```python
from build123d import *

# Parameters (mm, degrees)
SKETCH1_W            = 100
SKETCH1_H            = 40
BOSS_EXTRUDE1_DEPTH  = 150
CUT_EXTRUDE1_DEPTH   = 41
FILLET1_R            = 30
FILLET1_OF_MIRROR1_R = 30


with BuildPart() as part:
    # Sketch1 → Boss-Extrude1 (new body)
    with BuildSketch(Plane.XY):
        with Locations((-50, 20)):
            Rectangle(SKETCH1_W, SKETCH1_H)
    boss_extrude1 = extrude(amount=BOSS_EXTRUDE1_DEPTH)

    # Cut-Sweep1: sweep along a path in Sketch3
    with BuildLine(Plane(origin=(0, 40, 0), x_dir=(1, 0, 0), z_dir=(0, 1, 0))) as cut_sweep1_path:
        Line((-100, -127.5), (-55, -127.5))
        ThreePointArc((-55, -127.5), (-33.786796564, -118.713203436), (-25, -97.5))
        Line((-25, -97.5), (-25, -25))
    # Sketch2 → Cut-Sweep1 (sweep, cut)
    with BuildSketch(Plane.ZY.offset(100)):
        Polygon((135, 40), (120, 40), (120, 20), (112.5, 20), (112.5, 5), (142.5, 5), (142.5, 20), (135, 20), align=None)
    cut_sweep1 = sweep(path=cut_sweep1_path.line, mode=Mode.SUBTRACT)

    # Sketch4 → Cut-Extrude1 (cut, through all)
    with BuildSketch(Plane(origin=(0, 40, 0), x_dir=(1, 0, 0), z_dir=(0, 1, 0))):
        with BuildLine():
            Line((-52.5, -25), (-52.5, 0))
            Line((-52.5, 0), (-100, 0))
            Line((-100, 0), (-100, -100))
            Line((-100, -100), (-55, -100))
            ThreePointArc((-55, -100), (-53.232233047, -99.267766953), (-52.5, -97.5))
            Line((-52.5, -97.5), (-52.5, -25))
        make_face()
    cut_extrude1 = extrude(amount=-CUT_EXTRUDE1_DEPTH, mode=Mode.SUBTRACT)

    # Fillet1
    fillet1_edges = [part.edges().sort_by_distance(p)[0] for p in [
        (-52.5, 20, 0),
    ]]
    fillet(fillet1_edges, radius=FILLET1_R)

    # Mirror1: Boss-Extrude1, Cut-Sweep1, Cut-Extrude1 across plane
    add(boss_extrude1.mirror(Plane(origin=(0, 0, 150), x_dir=(0, 0, 1), z_dir=(-1, 0, 0))))
    add(cut_sweep1.mirror(Plane(origin=(0, 0, 150), x_dir=(0, 0, 1), z_dir=(-1, 0, 0))), mode=Mode.SUBTRACT)
    add(cut_extrude1.mirror(Plane(origin=(0, 0, 150), x_dir=(0, 0, 1), z_dir=(-1, 0, 0))), mode=Mode.SUBTRACT)

    # Fillet1 of Mirror1
    fillet1_of_mirror1_edges = [part.edges().sort_by_distance(p)[0] for p in [
        (52.5, 20, 0),
    ]]
    fillet(fillet1_of_mirror1_edges, radius=FILLET1_OF_MIRROR1_R)


solid = part.part
```
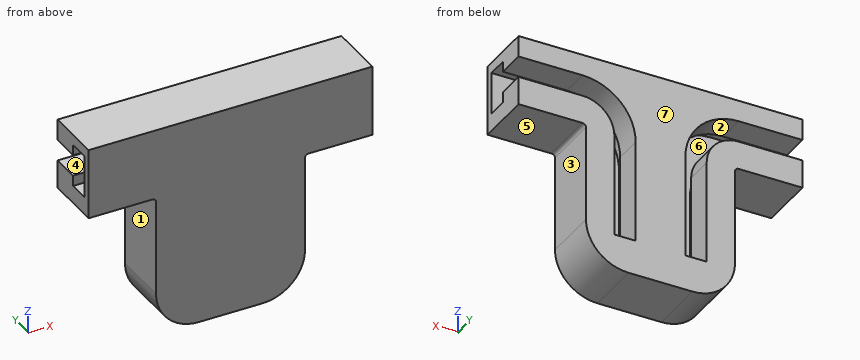
Could you check a few things on this model? Use its own coordinates, in mm. Face numbers are marked on the shaded views. A direction names the side the tool comes from. Round coordinates to 2 decimals unless told otherwise and drop trailing zeros. Loops run counter-clockwise (first coordinate to the right, second up) from the corner with the lowest first, then second, coordinate; pieces in that order, holes last. Notation, with made-up numbers: M 2,28.25 L 56,28.25 A24 ccw 56,62.25 Z; hole C 60,77 d1. An arc over 180 degrees is marked long. Write item = value, one per line.
1. I want a section at A-A, the plane z = 73.5. Write out the boundary of the cut face in (x, y), and give its area (3 significant figures).
Results below:
outline = M -52.5,0 L 52.5,0 L 52.5,40 L 32.5,40 L 32.5,20 L 40,20 L 40,5 L 10,5 L 10,20 L 17.5,20 L 17.5,40 L -17.5,40 L -17.5,20 L -10,20 L -10,5 L -40,5 L -40,20 L -32.5,20 L -32.5,40 L -52.5,40 Z
area = 2,700 mm²
2. Which directions (+Z, -Z, +X, -X, +Y, -Y) give clear straight access to the entire face, cutting with the end or side of a thin tool? Please do the marked faces 1, 2, 3 and 4.
Results below:
face_1 = -Z, -X, +Y, -Y
face_2 = +Y
face_3 = -Z, +X, +Y, -Y
face_4 = -X, +Y
3. I want a section at D-D, the plane y = 14.5. Write out the boundary of the cut face in (x, z), and give its area (3 significant figures).
Results below:
outline = M -100,100 L -55,100 A2.5 cw -52.5,97.5 L -52.5,30 A30 ccw -22.5,0 L 22.5,0 A30 ccw 52.5,30 L 52.5,97.5 A2.5 cw 55,100 L 100,100 L 100,112.5 L 55,112.5 A15 ccw 40,97.5 L 40,25 L 10,25 L 10,97.5 A45 cw 55,142.5 L 100,142.5 L 100,150 L -100,150 L -100,142.5 L -55,142.5 A45 cw -10,97.5 L -10,25 L -40,25 L -40,97.5 A15 ccw -55,112.5 L -100,112.5 Z
area = 10,200 mm²
4. Will these pins go through, and if not, where does the flat tip stop? P1, Ø8, axis at y = 19.5, z = 75.5, coming from the -X side; P2, Ø16, axis at y = 35, z = 53.5, coming from the +X side; P3, Ø6, axis at x = 70.5, y = 28, coming from the -Z side.
Results below:
P1 = -52.5
P2 = 52.5
P3 = 100
5. Thinking about a two-plate mould opening in Z: for the marked faces 5, 6 and 7, which applies, +Z half, -Z half, draft (parallel to the pull), parting line (faces both ways), or undercut?
Results below:
face_5 = -Z half
face_6 = undercut
face_7 = draft
6. I want a section at B-B, the plane x = 83. Write out the boundary of the cut face in (y, z), and give its area (3 significant figures).
Results below:
outline = M 0,100 L 40,100 L 40,120 L 20,120 L 20,112.5 L 5,112.5 L 5,142.5 L 20,142.5 L 20,135 L 40,135 L 40,150 L 0,150 Z
area = 1,250 mm²
7. I want a section at C-C, the plane y = 35. Write out the boundary of the cut face in (x, z), and give its area (3 significant figures).
Results below:
outline = M -100,100 L -55,100 A2.5 cw -52.5,97.5 L -52.5,30 A30 ccw -22.5,0 L 22.5,0 A30 ccw 52.5,30 L 52.5,97.5 A2.5 cw 55,100 L 100,100 L 100,120 L 55,120 A22.5 ccw 32.5,97.5 L 32.5,25 L 17.5,25 L 17.5,97.5 A37.5 cw 55,135 L 100,135 L 100,150 L -100,150 L -100,135 L -55,135 A37.5 cw -17.5,97.5 L -17.5,25 L -32.5,25 L -32.5,97.5 A22.5 ccw -55,120 L -100,120 Z
area = 15,200 mm²
8. I need wall thicknesses on probe 1 along X at (y, z) = (5.5, 98); probe 2 along X at (y, z) = (34.5, 93); probe 3 along Z at (x, y) = (84, 38.5). Which ranges of each line are inside material? Lowest first, please.
Results below:
probe_1 = -52.55 to -40.01, -10 to 10, 40.01 to 52.55
probe_2 = -52.5 to -32.5, -17.5 to 17.5, 32.5 to 52.5
probe_3 = 100 to 120, 135 to 150
